from build123d import *

# Parameters (mm, degrees)
SKETCH1_R           = 8
BOSS_EXTRUDE1_DEPTH = 3
SKETCH2_R           = 5
BOSS_EXTRUDE2_DEPTH = 14
SKETCH3_R           = 2.5
BOSS_EXTRUDE3_DEPTH = 10
SKETCH4_R           = 0.85
CUT_EXTRUDE1_DEPTH  = 7.5


with BuildPart() as part:
    # Sketch1 → Boss-Extrude1 (new body)
    with BuildSketch(Plane.XY):
        Circle(SKETCH1_R)
    extrude(amount=BOSS_EXTRUDE1_DEPTH)

    # Sketch2 → Boss-Extrude2 (add)
    with BuildSketch(Plane.XY.offset(3)):
        Circle(SKETCH2_R)
    extrude(amount=BOSS_EXTRUDE2_DEPTH)

    # Sketch3 → Boss-Extrude3 (add)
    with BuildSketch(Plane.XY.offset(17)):
        Circle(SKETCH3_R)
    extrude(amount=BOSS_EXTRUDE3_DEPTH)

    # Sketch4 → Cut-Extrude1 (cut, symmetric)
    with BuildSketch(Plane(origin=(0, 0, 0), x_dir=(1, 0, 0), z_dir=(0, 1, 0))):
        with Locations((0, -14)):
            Circle(SKETCH4_R)
    extrude(amount=CUT_EXTRUDE1_DEPTH, both=True, mode=Mode.SUBTRACT)


solid = part.part
CAD build for the part. Positions are in the model's coordinates, mm. A direction names the side the tool comes from. Give positions to 0.01 mm unless a question says otherwise; leave off trailing zeros. Loops run counter-clockwise (first coordinate to the right, second up) from the corner with the lowest first, then second, coordinate; pieces in that order, holes last. Notation, with made-up numbers: M -3.5,32 L 49.5,32 A11 ccw 49.5,51 Z; hole C -5.75,87 d5. An arc over 180 degrees is marked long. Answer in a Markdown table with one row per item. Add a question column.
Item 1: Probe probe 1 along Z at (x, y) = (0, -0.5); probe 2 along Z at (x, y) = (-2.5, 4); probe 3 along Z at (x, y) = (-4.5, -3). List the from-to ranges inside material, lowest first.
Item 2: Band-saw the part on C-C on z = 22.5. Give the cut face in (x, y).
Item 3: Drop flat-ended pins along their axis: P1, Ø4, axis at y = 3.5, z = 23.5, coming from the +X side; P2, Ø1, axis at x = 4.5, z = 4.5, coming from the +Y side; P3, Ø6, axis at x = 5.5, z = 16, coming from the +Y side. Give the stop position or say it passes through.
Item 4: Tool access for faces 4 (the face through (0, 0, 27)), 5 (the face through (-0.54, -2.44, 21.93)): list every direction of +Z, -Z, +X, -X, +Y, -Y with a clear straight run to the whole face (end or side of a thin tool).
Item 5: Mould opens along X. For faces 1 (the face through (-1.08, -4.88, 9.9)), 2 (the face through (2, -2, 17)), 3 (the face through (-0.111, 0.07, 13.157)) say: +X half, -X half, draft (parallel to the pull), parting line (faces both ways), or undercut.
Item 6: Band-saw the part on A-A on y = 0. Give the cut face in (x, z).
Item 7: Band-saw the part on D-D on x = 4. Give the cut face in (y, z).
Item 8: Band-saw the part on B-B on x = 0. Give the cut face in (y, z).
Reply:
| question | item | result |
|---|---|---|
| 1 | probe 1 | z = 0 to 13.15, 14.85 to 27 |
| 1 | probe 2 | z = 0 to 17 |
| 1 | probe 3 | z = 0 to 3 |
| 2 | outline | C 0,0 d5 |
| 3 | P1 | stops at x = 2 |
| 3 | P2 | stops at y = 3 |
| 3 | P3 | stops at y = 4.33 |
| 4 | face 4 | +Z, +X, -X, +Y, -Y |
| 4 | face 5 | +Z |
| 5 | face 1 | parting line |
| 5 | face 2 | draft |
| 5 | face 3 | undercut |
| 6 | outline | M -8,0 L 8,0 L 8,3 L 5,3 L 5,17 L 2.5,17 L 2.5,27 L -2.5,27 L -2.5,17 L -5,17 L -5,3 L -8,3 Z; hole C 0,14 d1.7 |
| 7 | outline | M -6.93,0 L 6.93,0 L 6.93,3 L 3,3 L 3,17 L -3,17 L -3,3 L -6.93,3 Z |
| 8 | outline | M -8,0 L 8,0 L 8,3 L 5,3 L 5,13.15 L -5,13.15 L -5,3 L -8,3 Z; M -5,14.85 L 5,14.85 L 5,17 L 2.5,17 L 2.5,27 L -2.5,27 L -2.5,17 L -5,17 Z |
